Verification items for this drawing (mm, ordinates from the low corner). A direction names the side the tool comes from. Round coordinates to 2 decimals unless told otherwise and drop trailing zeros. Loops run counter-clockwise (first coordinate to the right, second up) from the corner with the lowest first, then second, coordinate; pieces in that order, holes last. Notation, with made-up numbers: (25.5, 23.5) -> (29.5, 23.5) arc R22 ccw to (29.5, 29.5) -> close; hole circle Ø2 at (41.5, 47). An arc over 180 degrees is marked (long way). Use a Markdown table: item, result. Add a question column.
Q1. Sectioned sample at B-B, the plane x = 24.75. Enter the section's corners in (y, z) (1 decimal), then the cut area to 3 significant figures.
Q2. Release check for a two-part mould opening along Y. For the marked faces 1, 2, 3 and 4 record: released by +Y, released by -Y, zero draft, split by the parting line, or undercut.
Q3. Sectioned sample at A-A, the plane z = 4.5. Give the number of separate pieces and of enclosed holes in the cut face.
Q4. Set-up check for the marked faces 5 and 6: record each of +Z, -Z, +X, -X, +Y, -Y from which the full face is reachable in a straight line by a thin tool's end or side.
Q5. Sectioned sample at C-C, the plane y = 13.5. Enter the section's corners in (x, z) (1 decimal), then the cut area to 3 significant figures.
Q6. Gauge pin test, flat end, axial feed: P1, Ø2, axis at x = 11, y = 3.5, coming from the +Z side. Record the tip position at first contact, or that the pin passes through.
Q7. Sectioned sample at D-D, the plane x = 10.5. Enter the section's corners in (y, z) (1 decimal).
Q8. Material ranges on L1, parallel to X at y = 6.5, z = 7.5 (1 decimal); L2, parallel to Y at x = 14.25, z = 7.5; L3, parallel to X at y = 6.75, z = 2.25 (1 decimal), recorded low to high.
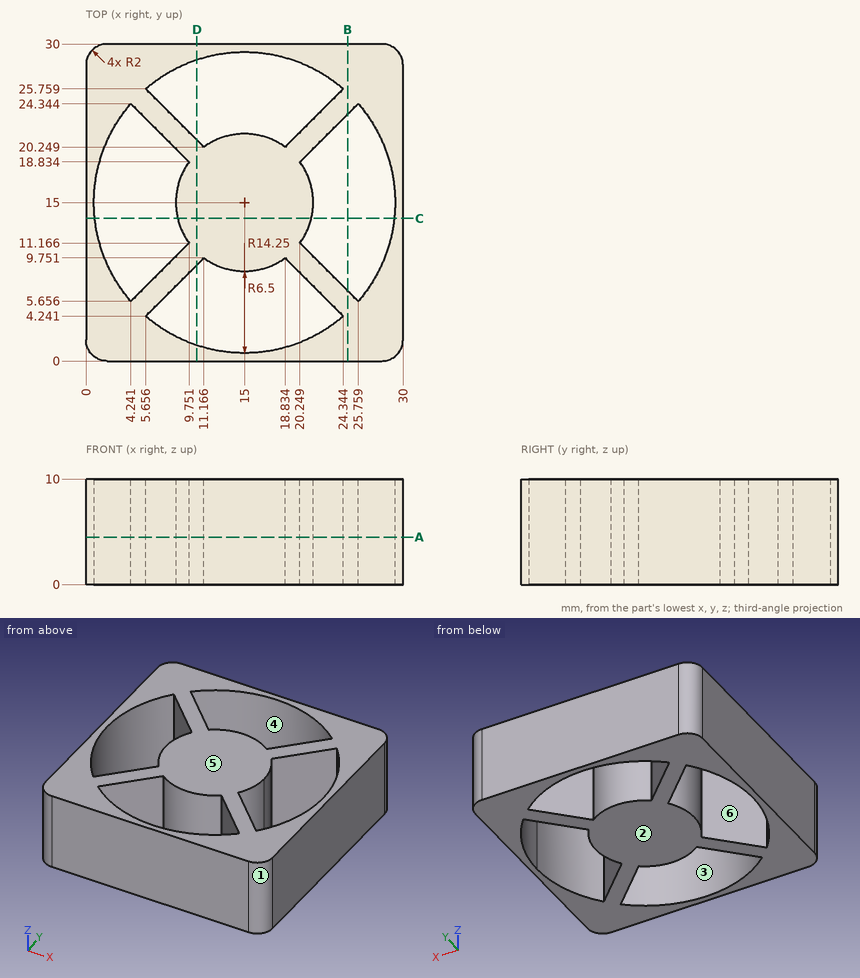
Values:
| question | item | result |
|---|---|---|
| 1 | outline | (0, 0) -> (6.7, 0) -> (6.7, 10) -> (0, 10) -> close; (23.3, 0) -> (30, 0) -> (30, 10) -> (23.3, 10) -> close |
| 1 | area | 133 mm^2 |
| 2 | face 1 | released by -Y |
| 2 | face 2 | zero draft |
| 2 | face 3 | undercut |
| 2 | face 4 | undercut |
| 3 | separate pieces | 1 |
| 3 | enclosed holes | 4 |
| 4 | face 5 | +Z, +X, -X, +Y, -Y |
| 4 | face 6 | +Z, -Z |
| 5 | outline | (0, 0) -> (0.8, 0) -> (0.8, 10) -> (0, 10) -> close; (8.7, 0) -> (21.3, 0) -> (21.3, 10) -> (8.7, 10) -> close; (29.2, 0) -> (30, 0) -> (30, 10) -> (29.2, 10) -> close |
| 5 | area | 143 mm^2 |
| 6 | P1 | through |
| 7 | outline | (0, 0) -> (1.5, 0) -> (1.5, 10) -> (0, 10) -> close; (9.1, 0) -> (20.9, 0) -> (20.9, 10) -> (9.1, 10) -> close; (28.5, 0) -> (30, 0) -> (30, 10) -> (28.5, 10) -> close |
| 8 | L1 | 0 to 3.6, 5.1 to 7.9, 22.1 to 24.9, 26.4 to 30 |
| 8 | L2 | 0 to 0.77, 8.54 to 21.46, 29.23 to 30 |
| 8 | L3 | 0 to 3.4, 5.3 to 8.2, 21.8 to 24.7, 26.6 to 30 |
